```python
from build123d import *

# Parameters (mm, degrees)
F0_R     = 57.15
F1_DEPTH = 9
F2_R     = 41.1777557501
F2_R_2   = 34.7361553424
F3_DEPTH = 7
F5_DEPTH = 7
F6_W     = 12
F6_H     = 6
F7_DEPTH = 9
F9_D     = 4.4958


with BuildPart() as f1:
    # F0 (on Top) → F1 (new body)
    with BuildSketch(Plane.XY):
        Circle(F0_R)
    extrude(amount=F1_DEPTH)

    # F2 (on face) → F3 (cut)
    with BuildSketch(Plane.XY.offset(9)):
        Circle(F2_R)
        Circle(F2_R_2, mode=Mode.SUBTRACT)
    extrude(amount=-F3_DEPTH, mode=Mode.SUBTRACT)

    # F4 (on face) → F5 (cut)
    with BuildSketch(Plane.XY.offset(9)):
        with BuildLine():
            ThreePointArc((9.2364512329, -4.5815780759), (10.0382703258, -2.3528743932), (10.3103292403, 0))
            ThreePointArc((10.3103292403, 0), (9.9709085428, 2.6237133751), (8.9749942157, 5.0746790905))
            Line((8.9749942157, 5.0746790905), (8.9749942157, -4.5815780759))
            Line((8.9749942157, -4.5815780759), (9.2364512329, -4.5815780759))
        make_face()
        with BuildLine():
            Line((37.7700850368, 5.0746790905), (34.3634707226, 5.0746790905))
            ThreePointArc((34.3634707226, 5.0746790905), (34.6428588969, 2.544172837), (34.7361553424, 0))
            ThreePointArc((34.7361553424, 0), (34.6602041198, -2.2958088649), (34.4326825895, -4.5815780759))
            Line((34.4326825895, -4.5815780759), (37.7700850368, -4.5815780759))
            Line((37.7700850368, -4.5815780759), (37.7700850368, 5.0746790905))
        make_face()
        with BuildLine():
            Line((8.9749942157, -4.5815780759), (8.9749942157, 5.0746790905))
            ThreePointArc((8.9749942157, 5.0746790905), (-10.3065518942, -0.27906468), (9.2364512329, -4.5815780759))
            Line((9.2364512329, -4.5815780759), (8.9749942157, -4.5815780759))
        make_face()
        with BuildLine():
            ThreePointArc((8.9749942157, 5.0746790905), (9.9709085428, 2.6237133751), (10.3103292403, 0))
            ThreePointArc((10.3103292403, 0), (10.0382703258, -2.3528743932), (9.2364512329, -4.5815780759))
            Line((9.2364512329, -4.5815780759), (34.4326825895, -4.5815780759))
            ThreePointArc((34.4326825895, -4.5815780759), (34.6602041198, -2.2958088649), (34.7361553424, 0))
            ThreePointArc((34.7361553424, 0), (34.6428588969, 2.544172837), (34.3634707226, 5.0746790905))
            Line((34.3634707226, 5.0746790905), (8.9749942157, 5.0746790905))
        make_face()
    extrude(amount=-F5_DEPTH, mode=Mode.SUBTRACT)

    # F6 (on face) → F7 (cut)
    with BuildSketch(Plane(origin=(0, 0, 0), x_dir=(1, 0, 0), z_dir=(0, 0, -1))):
        with Locations((30.4291332662, 33.5408807993)):
            Rectangle(F6_W, F6_H)
    extrude(amount=-F7_DEPTH, mode=Mode.SUBTRACT)

    # F9 (through all)
    with Locations(Plane.XY.offset(9)):
        with Locations((0, 49.4705886591), (-49.4705886591, 0), (0, -49.4705886591), (49.4705886591, 0)):
            Hole(F9_D / 2)


solid = f1.part
```
The listing builds one solid part. Answer for the finished solid, in the listing's coordinates (mm). A direction names the side the tool comes from. Round coordinates to 2 decimals unless told otherwise and drop trailing zeros. Loops run counter-clockwise (first coordinate to the right, second up) from the corner with the lowest first, then second, coordinate; pieces in that order, holes last.
1) Given P1, Ø2.5, axis at x = 29.5, z = 2.5, coming from the -Y side; P2, Ø1.8, axis at y = -34.5, z = 4, coming from the -X side; P3, Ø1.8, axis at y = -33.5, z = 4.5, coming from the +X side, each flat-ended and moving along its own axis, determine where each tip first touches the part or whether it passes through.
Outcome:
P1: stops at y = -49.68
P2: stops at x = -46.23
P3: stops at x = 46.94
2) A cutting plane is placed at C-C on z = 7. Determine the outline of the cut face in (x, y) (3 decimals).
Outcome:
outline: circle Ø114.3 at (0, 0); (8.975, 5.075) - (34.363, 5.075) arc R34.736 ccw (long way) to (34.433, -4.582) - (9.236, -4.582) arc R10.31 cw (long way) to start; hole circle Ø4.496 at (-49.471, 0); hole circle Ø4.496 at (0, -49.471); hole circle Ø4.496 at (0, 49.471); hole (24.429, -36.541) - (36.429, -36.541) - (36.429, -30.541) - (27.62, -30.541) arc R41.178 ccw (long way) to (24.429, -33.149) - close; hole circle Ø4.496 at (49.471, 0)
3) Consider line 1 (Y direction, x = 0, z = 5.25); line 2 (X direction, y = -36, z = 8.25); line 3 (Y direction, x = 6, z = 5.5). Determine where each line is inside the solid, lowest interval first.
Outcome:
line 1: y = -57.15 to -51.72, -47.22 to -41.18, -34.74 to -10.31, 10.31 to 34.74, 41.18 to 47.22, 51.72 to 57.15
line 2: x = -44.39 to -19.99, 19.99 to 24.43, 36.43 to 44.39
line 3: y = -56.83 to -40.74, -34.21 to -8.38, 8.38 to 34.21, 40.74 to 56.83
4) A cutting plane is placed at A-A on x = 0. Determine the outline of the cut face in (y, z).
Outcome:
outline: (-57.15, 0) - (-51.72, 0) - (-51.72, 9) - (-57.15, 9) - close; (-47.22, 0) - (47.22, 0) - (47.22, 9) - (41.18, 9) - (41.18, 2) - (34.74, 2) - (34.74, 9) - (10.31, 9) - (10.31, 2) - (-10.31, 2) - (-10.31, 9) - (-34.74, 9) - (-34.74, 2) - (-41.18, 2) - (-41.18, 9) - (-47.22, 9) - close; (51.72, 0) - (57.15, 0) - (57.15, 9) - (51.72, 9) - close
5) For a pull along X with two mould halves and no side action, classify faces 4 (the face through (38, 17, 9)), 5 (the face through (-51.547, -0.861, 4.437)), 6 (the face through (22, 5.075, 6)), 7 (the face through (-57.095, 2.513, 4.437)) as released by +X, released by -X, zero draft, split by the parting line, or undercut.
Outcome:
face 4: zero draft
face 5: undercut
face 6: undercut
face 7: split by the parting line
6) A cutting plane is placed at D-D on x = -50. Determine the outline of the cut face in (y, z).
Outcome:
outline: (-27.68, 0) - (-2.18, 0) - (-2.18, 9) - (-27.68, 9) - close; (2.18, 0) - (27.68, 0) - (27.68, 9) - (2.18, 9) - close
7) For faces 1 (the face through (-34.715, 1.211, 5.549)), 2 (the face through (-1, 1, 0)), 3 (the face through (36.429, -33, 4)), determine the directions among +Z, -Z, +X, -X, +Y, -Y from which every point of the face is accessible in a straight line to the end or side of a thin tool.
Outcome:
face 1: +Z
face 2: -Z, +X, -X, +Y, -Y
face 3: +Z, -Z
8) A cutting plane is placed at B-B on y = 0. Determine the outline of the cut face in (x, z).
Outcome:
outline: (-57.15, 0) - (-51.72, 0) - (-51.72, 9) - (-57.15, 9) - close; (-47.22, 0) - (47.22, 0) - (47.22, 9) - (41.18, 9) - (41.18, 2) - (-10.31, 2) - (-10.31, 9) - (-34.74, 9) - (-34.74, 2) - (-41.18, 2) - (-41.18, 9) - (-47.22, 9) - close; (51.72, 0) - (57.15, 0) - (57.15, 9) - (51.72, 9) - close
